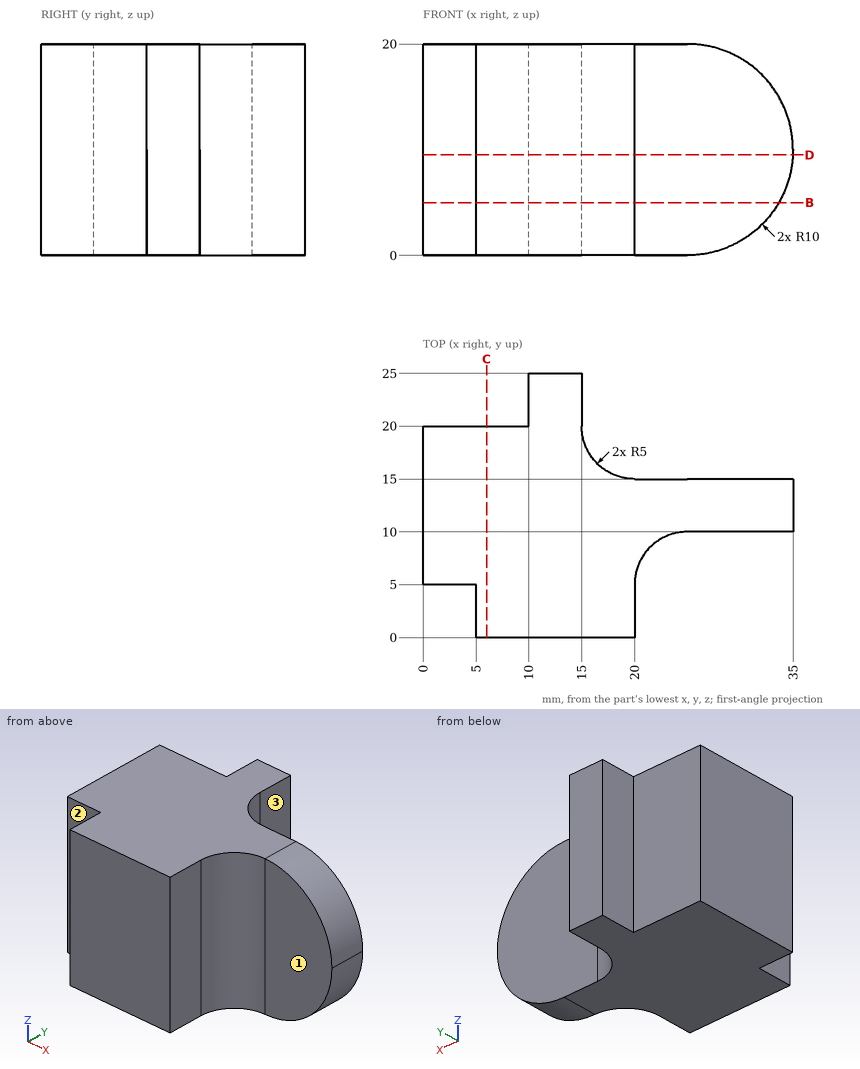
Input: dimensioned drawing with shaded views. Units: mm. Origin: part minimum x, y, z. A direction names the side the tool comes from. Coordinates: 2 decimals unless noted, no trailing zeros. Loops run counter-clockwise (first coordinate to the right, second up) from the corner with the lowest first, then second, coordinate; pieces in that order, holes last. Notation, with made-up numbers: M 57.5,58 L 69.5,58 A15 ccw 69.5,81 Z; hole C 5.25,8.5 d4. An arc over 180 degrees is marked long. Use a Markdown table: item, result. Add a question column.
Q1. Section query D-D, the plane z = 9.5. Return loops of the section in (x, y), and give its area (3 significant figures).
Q2. Material intervals for L1, parallel to Y at x = 4.5, z = 3; L2, parallel to Y at x = 27, z = 2.5, sorted ascending.
Q3. Section query C-C, the plane x = 6. Return loops of the section in (y, z).
Q4. Access query for the marked faces 1, 2 and 3. Directions: +Z, -Z, +X, -X, +Y, -Y. A direction counts if a zero-diameter tool reaches every point of the face in a straight line with its end or side. Return the directions, or none.
Q5. First-contact query: pin 1 (1.5 mm diameter, centred on y = 3.5, z = 13.5, fed in from +X); pin 2 (2.5 mm diameter, centred on y = 2, z = 6.5, fed in from -X); pin 3 (1.5 mm diameter, centred on y = 23, z = 8.5, fed in from +X). Flat tips, straight axial feed; report the tip coordinate or a pass-through.
Q6. Section query B-B, the plane z = 5. Return loops of the section in (x, y).
Result:
| question | item | result |
|---|---|---|
| 1 | outline | M 0,5 L 5,5 L 5,0 L 20,0 L 20,5 A5 cw 25,10 L 34.99,10 L 34.99,15 L 20,15 A5 cw 15,20 L 15,25 L 10,25 L 10,20 L 0,20 Z |
| 1 | area | 461 mm2 |
| 2 | L1 | y = 5 to 20 |
| 2 | L2 | y = 10 to 15 |
| 3 | outline | M 0,0 L 20,0 L 20,20 L 0,20 Z |
| 4 | face 1 | +Z, -Z, +X, -Y |
| 4 | face 2 | +Z, -Z, -X, -Y |
| 4 | face 3 | +Z, -Z, +X, +Y |
| 5 | pin 1 | stops at x = 20 |
| 5 | pin 2 | stops at x = 5 |
| 5 | pin 3 | stops at x = 15 |
| 6 | outline | M 0,5 L 5,5 L 5,0 L 20,0 L 20,5 A5 cw 25,10 L 33.66,10 L 33.66,15 L 20,15 A5 cw 15,20 L 15,25 L 10,25 L 10,20 L 0,20 Z |
